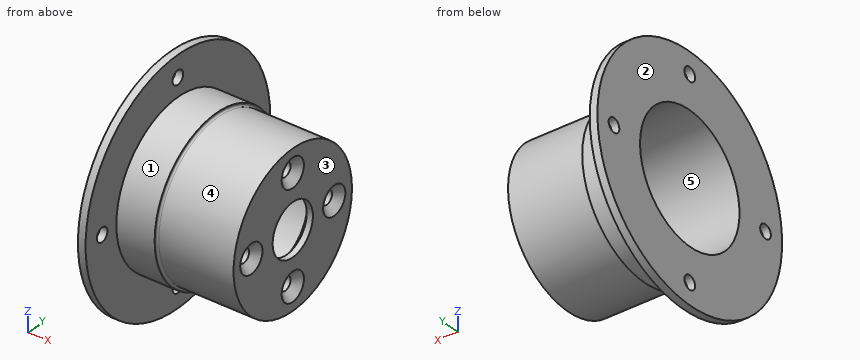
```python
from build123d import *

# Parameters (mm, degrees)
CSK_FOR_M4_FLAT_HEAD_MACHINE_SCREW1_D           = 4.5
CSK_FOR_M4_FLAT_HEAD_MACHINE_SCREW1_DEPTH       = 5
CSK_FOR_M4_FLAT_HEAD_MACHINE_SCREW1_CSINK_D     = 9.4
CSK_FOR_M4_FLAT_HEAD_MACHINE_SCREW1_CSINK_ANGLE = 90
FILLET1_R                                       = 0.6
M4_CLEARANCE_HOLE1_D                            = 4.5
M4_CLEARANCE_HOLE1_DEPTH                        = 2.5


with BuildPart() as part:
    # Sketch2 → Revolve1 (revolve)
    with BuildSketch(Plane.XY):
        Polygon((0, 21), (35, 21), (35, 12.75), (38, 12.75), (38, 8.5), (40, 8.5), (40, 25), (15, 25), (15, 26), (2.5, 26), (2.5, 39), (0, 39), (0, 26), align=None)
    revolve(axis=Axis((-64.103352454, 0, 0), (1, 0, 0)))

    # CSK for M4 Flat Head Machine Screw1
    with Locations(Plane(origin=(40, 0, 0), x_dir=(0, 0, -1), z_dir=(1, 0, 0))):
        with Locations((0, 17.5), (17.5, 0), (0, -17.5), (-17.5, 0)):
            CounterSinkHole(CSK_FOR_M4_FLAT_HEAD_MACHINE_SCREW1_D / 2, CSK_FOR_M4_FLAT_HEAD_MACHINE_SCREW1_CSINK_D / 2, depth=CSK_FOR_M4_FLAT_HEAD_MACHINE_SCREW1_DEPTH, counter_sink_angle=CSK_FOR_M4_FLAT_HEAD_MACHINE_SCREW1_CSINK_ANGLE)

    # Fillet1
    fillet1_edges = [part.edges().sort_by_distance(p)[0] for p in [
        (15, -25, 0),
    ]]
    fillet(fillet1_edges, radius=FILLET1_R)

    # M4 Clearance Hole1
    with Locations(Plane.ZY):
        with Locations((0, 32), (0, -32), (32, 0), (-32, 0)):
            Hole(M4_CLEARANCE_HOLE1_D / 2, depth=M4_CLEARANCE_HOLE1_DEPTH)


solid = part.part
```
Here's how the part is built. I have some questions about the finished solid (model axes, mm). Face numbers are marked on the shaded views. A direction names the side the tool comes from. Coordinates: 2 decimals unless noted, no trailing zeros. Order: outer loops, then holes, each group sorted by start corner. A loop starts at its lowest first (then second) coordinate and runs counter-clockwise, first axis right, second up.
Item 1: If we section it at B-B, the plane x = 4: List the corners of the cut face in (y, z) for me, then the cut area to 3 significant figures.
Response values:
outline: circle Ø52 at (0, 0); hole circle Ø42 at (0, 0)
area: 738 mm2
Item 2: I need wall thicknesses on probe 1 along Z at (x, y) = (35.9, 0); probe 2 along Z at (x, y) = (27, 0); probe 3 along X at (y, z) = (-31, 21). Which ranges of each line are inside material? Lowest first, please.
Response values:
probe 1: z = -25 to -19.75, -15.25 to -12.75, 12.75 to 15.25, 19.75 to 25
probe 2: z = -25 to -21, 21 to 25
probe 3: x = 0 to 2.5
Item 3: Thinking about a two-plate mould opening in Z: for the marked faces 3, 4 and 5, which applies, pulls with the +Z half, pulls with the -Z half, needs draft (parallel to the pull), parting line crosses it, or undercut?
Response values:
face 3: needs draft
face 4: parting line crosses it
face 5: undercut
Item 4: I'm going to push flat-ended pins straight in: pin 1 Ø5 at (y, z) = (-24, -2) entering from -X; pin 2 Ø12 at (x, y) = (27, -2) entering from -Z; pin 3 Ø6 at (y, z) = (0, 32) entering from +X; pin 4 Ø6 at (x, y) = (19.5, -16.5) entering from -Z. Where does each tip first touch, or does it pass through?
Response values:
pin 1: stops at x = 0
pin 2: stops at z = -25
pin 3: stops at x = 2.5
pin 4: stops at z = -21.04
Item 5: If we section it at C-C, the plane x = 30.5: List the corners of the cut face in (y, z) for me, then the cut area to 3 significant figures.
Response values:
outline: circle Ø50 at (0, 0); hole circle Ø42 at (0, 0)
area: 578 mm2
Item 6: If we section it at D-D, the plane y = -27.5: List the corners of the cut face in (x, z) for me, then the cut area to 3 significant figures.
Response values:
outline: (0, -27.65) - (2.5, -27.65) - (2.5, 27.65) - (0, 27.65) - close
area: 138 mm2
Item 7: Which directions (+Z, -Z, +X, -X, +Y, -Y) give clear straight access to the entire face, cutting with the end or side of a thin tool? Please do the marked faces 1 and 2.
Response values:
face 1: +X
face 2: +Z, -Z, -X, +Y, -Y
Item 8: If we section it at A-A, the plane z = 32: List the corners of the cut face in (x, y) for me, then the cut area to 3 significant figures.
Response values:
outline: (0, -22.29) - (2.5, -22.29) - (2.5, -2.25) - (0, -2.25) - close; (0, 2.25) - (2.5, 2.25) - (2.5, 22.29) - (0, 22.29) - close
area: 100 mm2
